For this review, take the finished solid that the model builds, in its own axes (mm). A direction names the side the tool comes from. Round coordinates to 2 decimals unless told otherwise and drop trailing zeros. Write each loop counter-clockwise with the first axis right and the second up, starting at its lowest first coordinate (ties: lowest second). Pieces come first, ordered by that corner, then holes. Notation, with made-up numbers: (-34, 41) - (14, 41) arc R23 ccw to (14, 77) - close; hole circle Ø11 at (36, 29). An arc over 180 degrees is marked (long way). One line per item, written item: value. Start each with the question number.
Q1. For probe 1 along Y at (x, z) = (0, 2); probe 2 along Z at (x, y) = (-3.75, 0.5); probe 3 along X at (y, z) = (0.25, 8.5), list the stretches that pass through material, from the lowest coordinate up.
Q2. Tool access review of faces 1 (the face through (-0.54, -2.44, 4.96)), 2 (the face through (-1.64, -1.26, 2.44)), 3 (the face through (3.448, -2.028, 2.098)): name each direction out of +Z, -Z, +X, -X, +Y, -Y from which nothing blocks a thin tool from reaching the whole face with its end or side.
Q3. Mouldability with a two-part tool opening along Y and no side actions: class faces 4 (the face through (-3, 0, 7)), 5 (the face through (0, 4, 2)), 6 (the face through (-1, -2, 4.4)) as +Y half, -Y half, draft (parallel to the pull), parting line (faces both ways), or undercut.
Q4. Add section B-B on z = 8.5. Write out the cut boundary in (x, y), and give its area (3 significant figures).
Q5. Add section A-A on z = 3.75. Write out the cut boundary in (x, y).
Q6. Clearance check with a flat-ended pin moving along its axis: pin 1 Ø3 at (x, y) = (1.5, 3) entering from +Z. State where the tip first meets the part, or that it passes through.
Solid Edge part; units mm, degrees
sketch "Sketch1" plane through (0, 0, 0) normal (0, 0, 1) x (1, 0, 0)
  circle A0 centre (0, 0) radius 4.6188
extrude "Protrusion1" add sketch "Sketch1" along normal blind 6
sketch "Sketch2" plane through (0, 0, 0) normal (0, 0, 1) x (1, 0, 0)
  arc A0 (2.3094, 4) -> (4.6188, 0) centre (0, 0) cw
  line L0 (4.6188, 0) -> (2.3094, 4)
extrude "ExtrudedCutout_1" cut sketch "Sketch2" along normal blind 6
pattern_circular "Pattern1" count 6 over 360 about axis through (0, 0, 0) along (0, 0, 1) of "ExtrudedCutout_1"
sketch "Sketch3" plane through (0, 0, 0) normal (0, -1, 0) x (1, 0, 0)
  line L0 (0, 0) -> (3, 0)
  line L1 (3, 0) -> (3, 7.5)
  arc A0 (3, 7.5) -> (0, 10.5) centre (0, 7.5) ccw
revolve "RevolvedProtrusion_1" add sketch "Sketch3" angle 360 about axis through (0, 0, 18.1) along (0, 0, -1)
sketch "Sketch4" plane through (0, 0, 0) normal (0, -1, 0) x (1, 0, 0)
  line L0 (0, 0) -> (2.067, 0)
  line L1 (2.067, 0) -> (2.067, 4.4001)
  line L2 (2.067, 4.4001) -> (2.5, 4.4001)
  line L3 (2.5, 4.4001) -> (2.5, 5.5001)
  line L4 (2.5, 5.5001) -> (0, 6.9435)
revolve "RevolvedCutout_1" cut sketch "Sketch4" angle 360 about axis through (0, 0, 12.9269) along (0, 0, -1)
sketch "Sketch5" plane through (0, 0, 0) normal (0, -1, 0) x (1, 0, 0)
  line L0 (3.3213, 6) -> (7.4285, 6)
  line L1 (7.4285, 6) -> (7.4285, 2.2762)
  line L2 (7.4285, 2.2762) -> (3.75, 4.4)
  line L3 (3.75, 4.4) -> (3.3213, 6)
  line L4 (3.999, 0) -> (7.4285, 1.98)
  line L5 (7.4285, 1.98) -> (7.4285, 0)
  line L6 (7.4285, 0) -> (3.999, 0)
revolve "RevolvedCutout_2" cut sketch "Sketch5" angle 360 about axis through (0, 0, 0) along (0, 0, 1)
fillet "Round_1" radius 0.32 2 edges at (-3.3213, 0, 6) (-3.75, 0, 4.4)
cosmetic_thread "Thread_1" thread depth 4.4
chamfer "Chamfer_1" distance 0.433 angle 45 1 edges at (-2.067, 0, 0)
sketch "Sketch6" plane through (0, 0, 0) normal (0, 0, -1) x (-1, 0, 0)
  circle A0 centre (0, 0) radius 1.75
extrude "Cutout6" cut sketch "Sketch6" against normal through all
properties part number "NK108" material "Stahl"
Result set:
1. probe 1: y = -4 to -2.07, 2.07 to 4
1. probe 2: z = 0 to 4.4
1. probe 3: x = -2.82 to -1.73, 1.73 to 2.82
2. face 1: none
2. face 2: -Z
2. face 3: +Z, -Z, +X, -Y
3. face 4: parting line
3. face 5: +Y half
3. face 6: undercut
4. outline: circle Ø5.66 at (0, 0); hole circle Ø3.5 at (0, 0)
4. area: 15.5 mm^2
5. outline: (-4.62, 0) - (-2.31, -4) - (2.31, -4) - (4.62, 0) - (2.31, 4) - (-2.31, 4) - close; hole circle Ø4.13 at (0, 0)
6. pin 1: stops at z = 9.86
